from build123d import *

# Parameters (mm, degrees)
EXTRUDE_1_DEPTH = 1.4


with BuildPart() as part:
    # Эскиз2 → Бобышка-Вытянуть1 (new, symmetric)
    with BuildSketch(Plane.XY):
        Polygon((-229.2, -3), (-114.2, -3), (-114.2, -1), (-111.4, -1), (-111.4, -3), (3.6, -3), (3.6, -1), (6.4, -1), (6.4, -3), (121.4, -3), (121.4, -1), (124.2, -1), (124.2, -3), (226.4, -3), (226.4, -1), (229.2, -1), (229.2, 3), (-229.2, 3), (-232, 3), (-232, 2), (-229.2, 2), (-229.2, 0), (-232, 0), (-232, -1), (-229.2, -1), align=None)
    extrude(amount=EXTRUDE_1_DEPTH, both=True)


solid = part.part
Source: CAD feature listing. Evaluate the final solid. Frame: model axes, mm. Round coordinates to 2 decimals unless told otherwise and drop trailing zeros. Loops run counter-clockwise (first coordinate to the right, second up) from the corner with the lowest first, then second, coordinate; pieces in that order, holes last.
Q1. First-contact query: P1, Ø1.4, axis at x = 228.5, z = -0.5, coming from the -Y side; P2, Ø0.6, axis at y = 1, z = -0.5, coming from the -X side; P3, Ø0.6, axis at y = -2, z = -0.5, coming from the +X side. Flat tips, straight axial feed; report the tip coordinate or a pass-through.
Q2. Section A-A, the plane y = -2.1. Return loops of the section in (x, z).
Q3. Ray query, line 1 (X direction, y = -2.7, z = 1.1); line 2 (Y direction, x = 5.5, z = 0.2); line 3 (X direction, y = 0.4, z = -0.9). Return the intervals inside material, ascending.
Solutions:
1. P1: stops at y = -1
1. P2: stops at x = -229.2
1. P3: stops at x = 226.4
2. outline: (-229.2, -1.4) - (-114.2, -1.4) - (-114.2, 1.4) - (-229.2, 1.4) - close; (-111.4, -1.4) - (3.6, -1.4) - (3.6, 1.4) - (-111.4, 1.4) - close; (6.4, -1.4) - (121.4, -1.4) - (121.4, 1.4) - (6.4, 1.4) - close; (124.2, -1.4) - (226.4, -1.4) - (226.4, 1.4) - (124.2, 1.4) - close
3. line 1: x = -229.2 to -114.2, -111.4 to 3.6, 6.4 to 121.4, 124.2 to 226.4
3. line 2: y = -1 to 3
3. line 3: x = -229.2 to 229.2
